from build123d import *

# Parameters (mm, degrees)
EXTRUDE_1_DEPTH     = 4
SKETCH_5_W          = 390
SKETCH_5_H          = 17
EXTRUDE_2_DEPTH     = 3
SKETCH_7_R          = 3.5
CUT_EXTRUDE_1_DEPTH = 407.957000186
SKETCH_8_W          = 340
SKETCH_8_H          = 3
EXTRUDE_3_DEPTH     = 13
SKETCH_9_W          = 14
SKETCH_9_H          = 17
CUT_EXTRUDE_2_DEPTH = 3
SKETCH_18_W         = 3
SKETCH_18_H         = 45
EXTRUDE_4_DEPTH     = 13
SKETCH_19_R         = 3
CUT_EXTRUDE_3_DEPTH = 13
SKETCH_20_R         = 3
CUT_EXTRUDE_4_DEPTH = 407.809537745
SKETCH_22_R         = 3
CUT_EXTRUDE_5_DEPTH = 13


with BuildPart() as part:
    # 草图1 → 凸台-拉伸1 (new body)
    with BuildSketch(Plane.XY):
        with BuildLine():
            Line((0, 0), (390, 0))
            Line((390, 0), (390, -90))
            ThreePointArc((390, -90), (382.67766953, -107.67766953), (365, -115))
            Line((365, -115), (25, -115))
            ThreePointArc((25, -115), (7.32233047, -107.67766953), (0, -90))
            Line((0, -90), (0, 0))
        make_face()
    extrude(amount=EXTRUDE_1_DEPTH)

    # 草图5 → 凸台-拉伸2 (add)
    with BuildSketch(Plane(origin=(0, 0, 0), x_dir=(1, 0, 0), z_dir=(0, 1, 0))):
        with Locations((195, 4.5)):
            Rectangle(SKETCH_5_W, SKETCH_5_H)
    extrude(amount=-EXTRUDE_2_DEPTH)

    # 草图7 → 切除-拉伸1 (cut, through all)
    with BuildSketch(Plane.XY.offset(4)):
        with Locations((167, -96.601136347)):
            Circle(SKETCH_7_R)
        with Locations((149.963903366, -39)):
            Circle(SKETCH_7_R)
        with Locations(Location((223, -96.601136347, 0), (0, 0, 180))):
            Circle(SKETCH_7_R)
        with Locations(Location((240.036096634, -39, 0), (0, 0, 180))):
            Circle(SKETCH_7_R)
        with BuildLine():
            ThreePointArc((168.147738424, -48.1103316), (195, -57), (221.852261576, -48.1103316))
            ThreePointArc((221.852261576, -48.1103316), (222.97574381, -47.716458908), (224.124012489, -48.030826634))
            ThreePointArc((224.124012489, -48.030826634), (230.355339059, -47.355339059), (231.030826634, -41.124012489))
            ThreePointArc((231.030826634, -41.124012489), (230.716458908, -39.97574381), (231.1103316, -38.852261576))
            ThreePointArc((231.1103316, -38.852261576), (195, 33), (158.8896684, -38.852261576))
            ThreePointArc((158.8896684, -38.852261576), (159.283541092, -39.97574381), (158.969173366, -41.124012489))
            ThreePointArc((158.969173366, -41.124012489), (159.644660941, -47.355339059), (165.875987511, -48.030826634))
            ThreePointArc((165.875987511, -48.030826634), (167.02425619, -47.716458908), (168.147738424, -48.1103316))
        make_face()
    extrude(amount=-CUT_EXTRUDE_1_DEPTH, mode=Mode.SUBTRACT)

    # 草图8 → 凸台-拉伸3 (add)
    with BuildSketch(Plane(origin=(0, 0, 0), x_dir=(-1, 0, 0), z_dir=(0, 0, -1))):
        with Locations((-195, -113.5)):
            Rectangle(SKETCH_8_W, SKETCH_8_H)
    extrude(amount=EXTRUDE_3_DEPTH)

    # 草图9 → 切除-拉伸2 (cut)
    with BuildSketch(Plane(origin=(0, 0, 0), x_dir=(1, 0, 0), z_dir=(0, 1, 0))):
        with Locations((383, 4.5)):
            Rectangle(SKETCH_9_W, SKETCH_9_H)
        with Locations((7, 4.5)):
            Rectangle(SKETCH_9_W, SKETCH_9_H)
    extrude(amount=-CUT_EXTRUDE_2_DEPTH, mode=Mode.SUBTRACT)

    # 草图18 → 凸台-拉伸4 (add)
    with BuildSketch(Plane(origin=(0, 0, 0), x_dir=(-1, 0, 0), z_dir=(0, 0, -1))):
        with Locations((-388.5, -33.5)):
            Rectangle(SKETCH_18_W, SKETCH_18_H)
        with Locations((-1.5, -33.5)):
            Rectangle(SKETCH_18_W, SKETCH_18_H)
    extrude(amount=EXTRUDE_4_DEPTH)

    # 草图19 → 切除-拉伸3 (cut)
    with BuildSketch(Plane(origin=(0, 0, 0), x_dir=(1, 0, 0), z_dir=(0, 1, 0))):
        with Locations(Location((270, 6, 0), (0, 0, 270))):
            Circle(SKETCH_19_R)
        with Locations(Location((350, 6, 0), (0, 0, 270))):
            Circle(SKETCH_19_R)
        with Locations(Location((40, 6, 0), (0, 0, 270))):
            Circle(SKETCH_19_R)
        with Locations(Location((120, 6, 0), (0, 0, 270))):
            Circle(SKETCH_19_R)
    extrude(amount=-CUT_EXTRUDE_3_DEPTH, mode=Mode.SUBTRACT)

    # 草图20 → 切除-拉伸4 (cut, through all)
    with BuildSketch(Plane(origin=(390, 0, 0), x_dir=(0, 0, -1), z_dir=(1, 0, 0))):
        with Locations(Location((6, -23, 0), (0, 0, 270))):
            Circle(SKETCH_20_R)
        with Locations(Location((6, -44, 0), (0, 0, 90))):
            Circle(SKETCH_20_R)
    extrude(amount=-CUT_EXTRUDE_4_DEPTH, mode=Mode.SUBTRACT)

    # 草图22 → 切除-拉伸5 (cut)
    with BuildSketch(Plane.XZ.offset(115)):
        with Locations((75, -6)):
            Circle(SKETCH_22_R)
        with Locations((135, -6)):
            Circle(SKETCH_22_R)
        with Locations((315, -6)):
            Circle(SKETCH_22_R)
        with Locations((255, -6)):
            Circle(SKETCH_22_R)
    extrude(amount=-CUT_EXTRUDE_5_DEPTH, mode=Mode.SUBTRACT)


solid = part.part
Input: part model. Units: mm. Frame: model coordinates. A direction names the side the tool comes from. Give positions to 0.01 mm unless a question says otherwise; leave off trailing zeros. Order: outer loops, then holes, each group sorted by start corner. A loop starts at its lowest first (then second) coordinate and runs counter-clockwise, first axis right, second up.
Q1. Ray query, probe 1 along Y at (x, z) = (321, -4); probe 2 along X at (y, z) = (-44.5, 3); probe 3 along Z at (x, y) = (389.35, -23). Return the intervals inside material, ascending.
Checked values:
probe 1: y = -115 to -112, -3 to 0
probe 2: x = 0 to 158.23, 231.77 to 390
probe 3: z = -13 to -9, -3 to 4
Q2. Section C-C on z = -6. State how many separate pieces and enclosed holes the cut face has, and give its area (3 significant figures).
Checked values:
separate pieces: 17
enclosed holes: 0
area: 1,900 mm2
Q3. Section D-D on x = 202. Output: boundary loops of the cut face in (y, z), and give its area (3 significant figures).
Checked values:
outline: (-115, -13) - (-112, -13) - (-112, 0) - (-56.45, 0) - (-56.45, 4) - (-115, 4) - close
area: 273 mm2
Q4. Contact query for flat-ended pins moving along their axis: pin 1 Ø4.5 at (x, z) = (380, 2) entering from +Y; pin 2 Ø2.5 at (y, z) = (-1, -8) entering from -X; pin 3 Ø5 at (x, y) = (148.5, -15) entering from -Z. Output: stop coordinate, or through.
Checked values:
pin 1: stops at y = -3
pin 2: stops at x = 14
pin 3: stops at z = 0
Q5. Draft query along Y for faces 4 (the cylindrical face through (153.302, -37.949, 2.028)), 5 (the cylindrical face through (382.871, -107.482, 1.972)), 6 (the flat face through (387, -34, -6)). Return one class per face: +Y half, -Y half, draft (parallel to the pull), parting line (faces both ways), or undercut.
Checked values:
face 4: undercut
face 5: -Y half
face 6: draft
Q6. Set-up query: faces 1 (the cylindrical face through (150.15, -15.67, 0.58)), 2 (the flat face through (3, -34, -6)), 3 (the flat face through (197, -112, -6)). Return all of +Z, -Z, +X, -X, +Y, -Y with unobstructed straight access to the full face (end or side cutting, diameter ignored); none if empty.
Checked values:
face 1: +Z, -Z
face 2: -Z, +Y, -Y
face 3: -Z, +X, -X
Q7. Section A-A on x = 323. Output: boundary loops of the cut face in (y, z).
Checked values:
outline: (-115, -13) - (-112, -13) - (-112, 0) - (-3, 0) - (-3, -13) - (0, -13) - (0, 4) - (-115, 4) - close
Q8. Section B-B on y = -62.5. Output: boundary loops of the cut face in (x, z).
Checked values:
outline: (0, 0) - (390, 0) - (390, 4) - (0, 4) - close
